```python
from build123d import *

# Parameters (mm, degrees)
F0_W                 = 70.5
F0_H                 = 70.5
F1_DEPTH             = 10
F2_W                 = 70.5
F2_H                 = 70.5
F3_DEPTH             = 10
F4_SIZE2             = 9.99999
F4_SIZE              = 35.24999
F5_W                 = 66.5
F5_H                 = 66.5
F6_DEPTH             = 8
F9_D                 = 3.4
F9_DEPTH             = 12
F9_CSINK_D           = 6.72
F9_CSINK_ANGLE       = 90
F9_TIP               = 1.0214630523
F9_ON_F8_D           = 3.4
F9_ON_F8_DEPTH       = 12
F9_ON_F8_CSINK_D     = 6.72
F9_ON_F8_CSINK_ANGLE = 90
F9_ON_F8_TIP         = 1.0214630523


# Not quite as in the source:
# - a fillet or chamfer is up to 0.001 mm smaller than in the source, because OpenCascade refuses the exact size


with BuildPart() as f1:
    # F0 (on Top) → F1 (new body)
    with BuildSketch(Plane.XY):
        with Locations((35.25, 35.25)):
            Rectangle(F0_W, F0_H)
    extrude(amount=F1_DEPTH)

    # F2 (on face) → F3 (join)
    with BuildSketch(Plane.XY.offset(10)):
        with Locations((35.25, 35.25)):
            Rectangle(F2_W, F2_H)
    extrude(amount=F3_DEPTH)

    # F4 (size 35.25 and 10 in the source; OpenCascade refuses exactly that, so slightly less here)
    f4_edges = [f1.edges().sort_by_distance(p)[0] for p in [
        (35.25, 70.5, 20),
        (0, 35.25, 20),
        (35.25, 0, 20),
        (70.5, 35.25, 20),
    ]]
    f4_side = f1.faces().sort_by_distance((35.25, 35.25, 20))[0]
    chamfer(f4_edges, length=F4_SIZE, length2=F4_SIZE2, reference=f4_side)

    # F5 (on face) → F6 (cut)
    with BuildSketch(Plane(origin=(0, 0, 0), x_dir=(1, 0, 0), z_dir=(0, 0, -1))):
        with Locations((35.25, -35.25)):
            Rectangle(F5_W, F5_H)
    extrude(amount=-F6_DEPTH, mode=Mode.SUBTRACT)

    # F9
    with Locations(Plane.XZ):
        with Locations((34.25, 5)):
            CounterSinkHole(F9_D / 2, F9_CSINK_D / 2, depth=F9_DEPTH, counter_sink_angle=F9_CSINK_ANGLE)
            with Locations((0, 0, -(F9_DEPTH + F9_TIP / 2))):  # 118° drill point
                Cone(0, F9_D / 2, F9_TIP, mode=Mode.SUBTRACT)

    # F9 on F8
    with Locations(Plane(origin=(0, 70.5, 0), x_dir=(-1, 0, 0), z_dir=(0, 1, 0))):
        with Locations((-34.25, 5)):
            CounterSinkHole(F9_ON_F8_D / 2, F9_ON_F8_CSINK_D / 2, depth=F9_ON_F8_DEPTH, counter_sink_angle=F9_ON_F8_CSINK_ANGLE)
            with Locations((0, 0, -(F9_ON_F8_DEPTH + F9_ON_F8_TIP / 2))):  # 118° drill point
                Cone(0, F9_ON_F8_D / 2, F9_ON_F8_TIP, mode=Mode.SUBTRACT)


solid = f1.part
```
Verification items for the finished model (mm, model axes). A direction names the side the tool comes from. Round coordinates to 2 decimals unless told otherwise and drop trailing zeros. Order: outer loops, then holes, each group sorted by start corner. A loop starts at its lowest first (then second) coordinate and runs counter-clockwise, first axis right, second up. Notation, with made-up numbers: (55.25, 58) - (97.25, 58) arc R19 cw to (97.25, 75) - close; hole circle Ø11 at (-4.5, 7.25). An arc over 180 degrees is marked (long way). Use CSV: the item, a comma, the result in double quotes. Start each with the question number.
1) Mould release check, pull along Y, two halves, no side actions. Record for faces 3 (the flat face through (32, 1, 0)), 4 (the flat face through (35, 68.5, 3)), 5 (the flat face through (34.8, 70.5, 0.5)): +Y half, -Y half, draft (parallel to the pull), parting line (faces both ways), or undercut.
2) Section check D-D, the plane x = 21. Record the cut outline in (y, z), plus the area to 3 significant figures.
3) Section check B-B, the plane x = 34.25. Record the cut outline in (y, z).
4) Go/stop test with flat-tipped pins: P1, Ø2, axis at x = 17, y = 29, coming from the +Z side; P2, Ø6, axis at x = 20, z = 12.5, coming from the +Y side; P3, Ø5.5, axis at x = 34.25, z = 5, coming from the -Y side; P4, Ø4, axis at x = 34.25, z = 5, coming from the -Y side. Record where each tip stops, or that it passes through.
5) Section check A-A, the plane z = 5. Record the cut outline in (x, y).
6) Access from +Z, -Z, +X, -X, +Y, -Y to the whole of each face (thin tool, end or side, straight path). Record for faces 1 (the flat face through (35, 35, 8)), 2 (the cylindrical face through (32.68, 1.83, 4.35)).
7) Section check C-C, the plane y = 46.5. Record the cut outline in (x, z).
8) Thickness scan on L1, parallel to X at y = 68.6, z = 5; L2, parallel to Y at x = 54, z = 4.5. Record the ranges inside material, lowest first.
Answers:
1,face 3,"draft"
1,face 4,"undercut"
1,face 5,"+Y half"
2,outline,"(0, 0) - (2, 0) - (2, 8) - (68.5, 8) - (68.5, 0) - (70.5, 0) - (70.5, 10) - (49.5, 15.96) - (21, 15.96) - (0, 10) - close"
2,area,"468 mm²"
3,outline,"(0, 0) - (2, 0) - (2, 3.3) - (1.66, 3.3) - (0, 1.64) - close; (0, 8.36) - (1.66, 6.7) - (2, 6.7) - (2, 8) - (68.5, 8) - (68.5, 6.7) - (68.84, 6.7) - (70.5, 8.36) - (70.5, 10) - (36.25, 19.72) - (34.25, 19.72) - (0, 10) - close; (68.5, 0) - (70.5, 0) - (70.5, 1.64) - (68.84, 3.3) - (68.5, 3.3) - close"
4,P1,"stops at z = 15.11"
4,P2,"stops at y = 70.5"
4,P3,"stops at y = 0.61"
4,P4,"stops at y = 1.36"
5,outline,"(0, 0) - (30.89, 0) - (32.55, 1.66) - (32.55, 2) - (2, 2) - (2, 68.5) - (32.55, 68.5) - (32.55, 68.84) - (30.89, 70.5) - (0, 70.5) - close; (35.95, 1.66) - (37.61, 0) - (70.5, 0) - (70.5, 70.5) - (37.61, 70.5) - (35.95, 68.84) - (35.95, 68.5) - (68.5, 68.5) - (68.5, 2) - (35.95, 2) - close"
6,face 1,"-Z"
6,face 2,"+Y, -Y"
7,outline,"(0, 0) - (2, 0) - (2, 8) - (68.5, 8) - (68.5, 0) - (70.5, 0) - (70.5, 10) - (46.5, 16.81) - (24, 16.81) - (0, 10) - close"
8,L1,"x = 0 to 32.55, 35.95 to 70.5"
8,L2,"y = 0 to 2, 68.5 to 70.5"
